CAD build for the part. Positions are in the model's coordinates, mm. A direction names the side the tool comes from. Give positions to 0.01 mm unless a question says otherwise; leave off trailing zeros. Loops run counter-clockwise (first coordinate to the right, second up) from the corner with the lowest first, then second, coordinate; pieces in that order, holes last. Notation, with made-up numbers: M 43,-28.75 L 101,-28.75 A21 cw 101,-20.75 Z; hole C 73,78 d5. An arc over 180 degrees is marked long. Answer as CSV lines item,"result".
from build123d import *

# Parameters (mm, degrees)
SKETCH1_R           = 23
BOSS_EXTRUDE1_DEPTH = 10
FILLET1_R           = 0.8
SKETCH2_R           = 1.5
CUT_EXTRUDE1_DEPTH  = 6


with BuildPart() as part:
    # Sketch1 → Boss-Extrude1 (new body)
    with BuildSketch(Plane(origin=(0, 0, 0), x_dir=(1, 0, 0), z_dir=(0, 1, 0))):
        with Locations(Location((0, 0, 0), (0, 0, 270))):
            Circle(SKETCH1_R)
        with BuildLine():
            Line((-1, 21.977260976), (-1, 2.828427125))
            ThreePointArc((-1, 2.828427125), (-2.121320344, 2.121320344), (-2.828427125, 1))
            Line((-2.828427125, 1), (-21.977260976, 1))
            ThreePointArc((-21.977260976, 1), (-15.556349186, 15.556349186), (-1, 21.977260976))
        make_face(mode=Mode.SUBTRACT)
        with BuildLine():
            Line((1, 21.977260976), (1, 2.828427125))
            ThreePointArc((1, 2.828427125), (2.121320344, 2.121320344), (2.828427125, 1))
            Line((2.828427125, 1), (21.977260976, 1))
            ThreePointArc((21.977260976, 1), (15.556349186, 15.556349186), (1, 21.977260976))
        make_face(mode=Mode.SUBTRACT)
        with BuildLine():
            Line((-21.977260976, -1), (-2.828427125, -1))
            ThreePointArc((-2.828427125, -1), (-2.121320344, -2.121320344), (-1, -2.828427125))
            Line((-1, -2.828427125), (-1, -21.977260976))
            ThreePointArc((-1, -21.977260976), (-15.556349186, -15.556349186), (-21.977260976, -1))
        make_face(mode=Mode.SUBTRACT)
        with BuildLine():
            Line((1, -2.828427125), (1, -21.977260976))
            ThreePointArc((1, -21.977260976), (15.556349186, -15.556349186), (21.977260976, -1))
            Line((21.977260976, -1), (2.828427125, -1))
            ThreePointArc((2.828427125, -1), (2.121320344, -2.121320344), (1, -2.828427125))
        make_face(mode=Mode.SUBTRACT)
    extrude(amount=BOSS_EXTRUDE1_DEPTH)

    # Fillet1
    fillet1_edges = [part.edges().sort_by_distance(p)[0] for p in [
        (2.121320344, 10, -2.121320344),
        (12.40284405, 10, -1),
        (-2.121320344, 10, 2.121320344),
        (-12.40284405, 10, 1),
        (-1, 10, 12.40284405),
        (12.40284405, 10, 1),
        (2.121320344, 10, 2.121320344),
        (1, 10, 12.40284405),
        (-12.40284405, 10, -1),
        (-2.121320344, 10, -2.121320344),
        (-1, 10, -12.40284405),
        (1, 10, -12.40284405),
    ]]
    fillet(fillet1_edges, radius=FILLET1_R)

    # Sketch2 → Cut-Extrude1 (cut)
    with BuildSketch(Plane.XZ):
        with Locations(Location((0, 0, 0), (0, 0, 270))):
            Circle(SKETCH2_R)
    extrude(amount=-CUT_EXTRUDE1_DEPTH, mode=Mode.SUBTRACT)


solid = part.part
1) Mould opens along Z. For faces 1 (the face through (-2, 10, 0)), 2 (the face through (19.394, 4.93, 12.365)), 3 (the face through (0, 6, 0)) say: +Z half, -Z half, draft (parallel to the pull), parting line (faces both ways), or undercut.
Answer below:
face 1,"draft"
face 2,"parting line"
face 3,"undercut"
2) Band-saw the part on B-B on x = 8. Give the cut face in (y, z).
Answer below:
outline,"M 0,-21.56 L 10,-21.56 L 10,-20.49 L 0,-20.49 Z; M 0,-1 L 9.2,-1 A0.8 ccw 10,-0.2 L 10,0.2 A0.8 ccw 9.2,1 L 0,1 Z; M 0,20.49 L 10,20.49 L 10,21.56 L 0,21.56 Z"
3) Which spindle directions (+Z, -Z, +X, -X, +Y, -Y) get a long thin tool onto all of the face, cutting with end or side? Do faces 4 (the face through (-13, 5, 1)), 5 (the face through (0.45, 2.96, -1.43)), 6 (the face through (0, 0, 2)). Say none if no direction does.
Answer below:
face 4,"+Y, -Y"
face 5,"-Y"
face 6,"+Z, -Z, +X, -X, -Y"
4) Band-saw the part on A-A on y = 8.25. Give the cut face in (x, z).
Answer below:
outline,"C 0,0 d46; hole M -21.98,-1 A22 ccw -1,-21.98 L -1,-2.83 A3 cw -2.83,-1 Z; hole M -21.98,1 L -2.83,1 A3 cw -1,2.83 L -1,21.98 A22 ccw Z; hole M 1,-21.98 A22 ccw 21.98,-1 L 2.83,-1 A3 cw 1,-2.83 Z; hole M 1,2.83 A3 cw 2.83,1 L 21.98,1 A22 ccw 1,21.98 Z"
5) Band-saw the part on C-C on z = 15. Give the cut face in (x, y), and give its area (3 significant figures).
Answer below:
outline,"M -17.44,0 L -16.09,0 L -16.09,10 L -17.44,10 Z; M -1,0 L 1,0 L 1,9.2 A0.8 ccw 0.2,10 L -0.2,10 A0.8 ccw -1,9.2 Z; M 16.09,0 L 17.44,0 L 17.44,10 L 16.09,10 Z"
area,"46.6 mm^2"
6) Flat gauge pins, fed straight in: pin 1 (1.5 mm diameter, centred on y = 6, z = 16, fed in from -X); pin 2 (6 mm diameter, centred on x = -14, z = -12, fed in from -Y); pin 3 (5 mm diameter, centred on x = -17.5, y = 5.5, fed in from +Z); pin 4 (1.5 mm diameter, centred on y = 6.5, z = -1.5, fed in from -X). Where does each tip first touch, or does it go through?
Answer below:
pin 1,"stops at x = -17.22"
pin 2,"passes through"
pin 3,"stops at z = 17.44"
pin 4,"stops at x = -22.99"
7) Drill centre lines: line 1 (X direction, y = 1.9, z = 0); line 2 (X direction, y = 3.25, z = 6); line 3 (Z direction, x = -8.5, y = 8.25). Where is each one in solid material? Low to high. Write a range as from..to.
Answer below:
line 1,"x = -23..-1.5, 1.5..23"
line 2,"x = -22.2..-21.17, -1..1, 21.17..22.2"
line 3,"z = -21.37..-20.29, -1..1, 20.29..21.37"
